from build123d import *

# Parameters (mm, degrees)
SKETCH1_W           = 40
SKETCH1_H           = 40
BOSS_EXTRUDE1_DEPTH = 8
SKETCH2_R           = 1.7
CUT_EXTRUDE1_DEPTH  = 58.131427428
SKETCH3_R           = 1.25
CUT_EXTRUDE2_DEPTH  = 58.131427428
SKETCH4_R           = 2.9
CUT_EXTRUDE3_DEPTH  = 3.2
CHAMFER1_SIZE       = 3.536
CHAMFER2_SIZE       = 0.5


with BuildPart() as part:
    # Sketch1 → Boss-Extrude1 (new body)
    with BuildSketch(Plane.XY):
        with Locations((20, 20)):
            Rectangle(SKETCH1_W, SKETCH1_H)
    extrude(amount=BOSS_EXTRUDE1_DEPTH)

    # Sketch2 → Cut-Extrude1 (cut, through all)
    with BuildSketch(Plane.XY.offset(8)):
        with Locations((5, 35)):
            Circle(SKETCH2_R)
        with Locations((35, 35)):
            Circle(SKETCH2_R)
        with Locations((5, 5)):
            Circle(SKETCH2_R)
        with Locations((35, 5)):
            Circle(SKETCH2_R)
    extrude(amount=-CUT_EXTRUDE1_DEPTH, mode=Mode.SUBTRACT)

    # Sketch3 → Cut-Extrude2 (cut, through all)
    with BuildSketch(Plane.XY.offset(8)):
        with Locations((17.66557685, 23.464101615)):
            Circle(SKETCH3_R)
        with Locations((21.66557685, 16.535898385)):
            Circle(SKETCH3_R)
    extrude(amount=-CUT_EXTRUDE2_DEPTH, mode=Mode.SUBTRACT)

    # Sketch4 → Cut-Extrude3 (cut)
    with BuildSketch(Plane.XY.offset(8)):
        with Locations((5, 35)):
            Circle(SKETCH4_R)
        with Locations((35, 35)):
            Circle(SKETCH4_R)
        with Locations((5, 5)):
            Circle(SKETCH4_R)
        with Locations((35, 5)):
            Circle(SKETCH4_R)
    extrude(amount=-CUT_EXTRUDE3_DEPTH, mode=Mode.SUBTRACT)

    # Chamfer1
    chamfer1_edges = [part.edges().sort_by_distance(p)[0] for p in [
        (0, 40, 4),
        (40, 40, 4),
        (40, 0, 4),
        (0, 0, 4),
    ]]
    chamfer(chamfer1_edges, length=CHAMFER1_SIZE)

    # Chamfer2
    chamfer2_edges = [part.edges().sort_by_distance(p)[0] for p in [
        (33.3, 35, 0),
        (3.3, 5, 0),
        (33.3, 5, 0),
        (3.3, 35, 0),
        (16.41557685, 23.464101615, 0),
        (16.41557685, 23.464101615, 8),
        (20.41557685, 16.535898385, 0),
        (20.41557685, 16.535898385, 8),
        (32.1, 35, 8),
        (33.3, 35, 4.8),
        (2.1, 5, 8),
        (3.3, 5, 4.8),
        (32.1, 5, 8),
        (33.3, 5, 4.8),
        (2.1, 35, 8),
        (3.3, 35, 4.8),
        (0, 20, 0),
        (0, 20, 8),
        (20, 40, 0),
        (40, 20, 0),
        (20, 0, 0),
        (1.768, 1.768, 0),
        (38.232, 1.768, 0),
        (38.232, 38.232, 0),
        (1.768, 38.232, 0),
        (20, 40, 8),
        (20, 0, 8),
        (40, 20, 8),
        (1.768, 1.768, 8),
        (38.232, 1.768, 8),
        (38.232, 38.232, 8),
        (1.768, 38.232, 8),
    ]]
    chamfer(chamfer2_edges, length=CHAMFER2_SIZE)


solid = part.part
Check sheet for the modelled part. Datum: model origin and axes. Units: mm. A direction names the side the tool comes from. Coordinates: 2 decimals unless noted, no trailing zeros. Write each loop counter-clockwise with the first axis right and the second up, starting at its lowest first coordinate (ties: lowest second). Pieces come first, ordered by that corner, then holes. Notation, with made-up numbers: M 59,81 L 95,81 A22 cw 95,91 Z; hole C 48.25,79.5 d5. An arc over 180 degrees is marked long. Answer as CSV lines item,"result".
Q1. Material ranges on probe 1 along Y at (x, z) = (5, 3.55); probe 2 along Y at (x, z) = (35, 6.3); probe 3 along Y at (x, z) = (17.5, 7.25), recorded low to high. Write a range as from..to.
Check result:
probe 1,"0..3.3, 6.7..33.3, 36.7..40"
probe 2,"0..2.1, 7.9..32.1, 37.9..40"
probe 3,"0..22.23, 24.7..40"
Q2. Set-up check for faces 1 (the face through (1.92, 1.97, 7.75)), 2 (the face through (34.1, 7.2, 4.8)): record each of +Z, -Z, +X, -X, +Y, -Y from which the full face is reachable in a straight line by a thin tool's end or side.
Check result:
face 1,"+Z, -X, -Y"
face 2,"+Z"
Q3. Cross-section at A-A (y = 5). Count the separate pieces of the cut face and the enclosed holes in it, then the cut area to 3 significant figures.
Check result:
separate pieces,"3"
enclosed holes,"0"
area,"248 mm^2"
Q4. Cross-section at C-C (z = 6.75). Record the boundary of the cut face in (x, y).
Check result:
outline,"M 0,3.54 L 3.54,0 L 36.46,0 L 40,3.54 L 40,36.46 L 36.46,40 L 3.54,40 L 0,36.46 Z; hole C 5,5 d5.8; hole C 5,35 d5.8; hole C 17.67,23.46 d2.5; hole C 21.67,16.54 d2.5; hole C 35,5 d5.8; hole C 35,35 d5.8"
Q5. Go/stop test with flat-tipped pins: pin 1 (1.7 mm diameter, centred on x = 3.5, y = 35.5, fed in from +Z); pin 2 (3.5 mm diameter, centred on x = 5, y = 35, fed in from -Z); pin 3 (3 mm diameter, centred on x = 17.67, y = 23.46, fed in from +Z). Record where each tip stops, or that it passes through.
Check result:
pin 1,"z = 4.8"
pin 2,"z = 0.45"
pin 3,"z = 7.76"
Q6. Cross-section at D-D (z = 2.25). Record the boundary of the cut face in (x, y), then the cut area to 3 significant figures.
Check result:
outline,"M 0,3.54 L 3.54,0 L 36.46,0 L 40,3.54 L 40,36.46 L 36.46,40 L 3.54,40 L 0,36.46 Z; hole C 5,5 d3.4; hole C 5,35 d3.4; hole C 17.67,23.46 d2.5; hole C 21.67,16.54 d2.5; hole C 35,5 d3.4; hole C 35,35 d3.4"
area,"1,530 mm^2"
Q7. Mould release check, pull along X, two halves, no side actions. Record for faces 3 (the face through (1.793, 38.257, 3.951)), 4 (the face through (17.395, 22.244, 4.049)), 5 (the face through (33.65, 3.97, 2.43)), 6 (the face through (20, 20, 0)): released by +X, released by -X, zero draft, split by the parting line, or undercut.
Check result:
face 3,"released by -X"
face 4,"undercut"
face 5,"undercut"
face 6,"zero draft"
